```python
from build123d import *

# Parameters (mm, degrees)
ESQUISSE4_R           = 1.5
EXTRUSION3_DEPTH      = 25
ESQUISSE5_OUTSIDE_W   = 153.718
ESQUISSE5_OUTSIDE_H   = 153.718
ESQUISSE5_OUTSIDE_W_2 = 71
ESQUISSE5_OUTSIDE_H_2 = 48
EXTRUSION4_DEPTH      = 13
ESQUISSE6_R           = 2
EXTRUSION5_DEPTH      = 10
ESQUISSE7_R           = 2
EXTRUSION6_DEPTH      = 10


with BuildPart() as part:
    # Esquisse1 → Révolution1 (revolve)
    with BuildSketch(Plane.XY):
        Polygon((19, -12), (59, -12), (59, 0), (15, 0), (15, -20), (9, -20), (9, -24), (19, -24), align=None)
    revolve(axis=Axis((0, 0, 0), (0, -1, 0)))

    # Esquisse4 → Extrusion3 (cut, through all)
    with BuildSketch(Plane.XZ.offset(24)):
        with Locations((0, 13)):
            Circle(ESQUISSE4_R)
        with Locations((13, 0)):
            Circle(ESQUISSE4_R)
        with Locations((0, -13)):
            Circle(ESQUISSE4_R)
        with Locations((-13, 0)):
            Circle(ESQUISSE4_R)
    extrude(amount=-EXTRUSION3_DEPTH, mode=Mode.SUBTRACT)

    # Esquisse5 outside → Extrusion4 (cut, through all)
    with BuildSketch(Plane.XZ.offset(12)):
        Rectangle(ESQUISSE5_OUTSIDE_W, ESQUISSE5_OUTSIDE_H)
        Rectangle(ESQUISSE5_OUTSIDE_W_2, ESQUISSE5_OUTSIDE_H_2, mode=Mode.SUBTRACT)
    extrude(amount=-EXTRUSION4_DEPTH, mode=Mode.SUBTRACT)

    # Esquisse6 → Extrusion5 (cut)
    with BuildSketch(Plane(origin=(35.5, 0, 0), x_dir=(0, 0, -1), z_dir=(1, 0, 0))):
        with Locations((-15, -6)):
            Circle(ESQUISSE6_R)
        with Locations((15, -6)):
            Circle(ESQUISSE6_R)
    extrude(amount=-EXTRUSION5_DEPTH, mode=Mode.SUBTRACT)

    # Esquisse7 → Extrusion6 (cut)
    with BuildSketch(Plane.ZY.offset(35.5)):
        with Locations((15, -6)):
            Circle(ESQUISSE7_R)
        with Locations((-15, -6)):
            Circle(ESQUISSE7_R)
    extrude(amount=-EXTRUSION6_DEPTH, mode=Mode.SUBTRACT)


solid = part.part
```
The model under review builds one solid part; all positions refer to its coordinate system, in mm. A direction names the side the tool comes from. Round coordinates to 2 decimals unless told otherwise and drop trailing zeros. Order: outer loops, then holes, each group sorted by start corner. A loop starts at its lowest first (then second) coordinate and runs counter-clockwise, first axis right, second up. Notation, with made-up numbers: (31, 55) -> (73, 55) arc R18 cw to (73, 73) -> close; hole circle Ø4 at (-4, 28.5). An arc over 180 degrees is marked (long way). Use a Markdown table: item, result.
Q1. We need section B-B on x = -13. Write out the cut boundary in (y, z), then the cut area to 3 significant figures.
Values:
| item | result |
|---|---|
| outline | (-24, -13.86) -> (-12, -13.86) -> (-12, -24) -> (0, -24) -> (0, -7.48) -> (-20, -7.48) -> (-20, -1.5) -> (-24, -1.5) -> close; (-24, 1.5) -> (-20, 1.5) -> (-20, 7.48) -> (0, 7.48) -> (0, 24) -> (-12, 24) -> (-12, 13.86) -> (-24, 13.86) -> close |
| area | 597 mm^2 |
Q2. We need section A-A on y = -6. Write out the cut boundary in (x, z), then the cut area to 3 significant figures.
Values:
| item | result |
|---|---|
| outline | (-35.5, -24) -> (35.5, -24) -> (35.5, -17) -> (25.5, -17) -> (25.5, -13) -> (35.5, -13) -> (35.5, 13) -> (25.5, 13) -> (25.5, 17) -> (35.5, 17) -> (35.5, 24) -> (-35.5, 24) -> (-35.5, 17) -> (-25.5, 17) -> (-25.5, 13) -> (-35.5, 13) -> (-35.5, -13) -> (-25.5, -13) -> (-25.5, -17) -> (-35.5, -17) -> close; hole circle Ø30 at (0, 0) |
| area | 2,540 mm^2 |
Q3. We need section C-C on z = 20.5. Write out the cut boundary in (x, y), then the cut area to 3 significant figures.
Values:
| item | result |
|---|---|
| outline | (-35.5, -12) -> (35.5, -12) -> (35.5, 0) -> (-35.5, 0) -> close |
| area | 852 mm^2 |
Q4. Mouldability with a two-part tool opening along Z and no side actions: class faces 1 (the cylindrical face through (-0.325, -22.028, 11.536)), 2 (the cylindrical face through (30.6, -7.2, 16.6)), 3 (the flat face through (-35.5, -6, 0)), 4 (the cylindrical face through (8.767, -17.916, -16.856)) as +Z half, -Z half, draft (parallel to the pull), parting line (faces both ways), or undercut.
Values:
| item | result |
|---|---|
| face 1 | undercut |
| face 2 | undercut |
| face 3 | draft |
| face 4 | parting line |
Q5. For line 1 (Z direction, x = 0, y = -22.35); line 2 (Z direction, x = 0, y = -14.5); line 3 (Y direction, x = 9, z = 6.5), list the stretches that pass through material, from the lowest coordinate up.
Values:
| item | result |
|---|---|
| line 1 | z = -19 to -14.5, -11.5 to -9, 9 to 11.5, 14.5 to 19 |
| line 2 | z = -19 to -15, 15 to 19 |
| line 3 | y = -24 to -20 |
Q6. We need section D-D on y = -11. Write out the cut boundary in (x, z).
Values:
| item | result |
|---|---|
| outline | (-35.5, -24) -> (35.5, -24) -> (35.5, 24) -> (-35.5, 24) -> close; hole circle Ø30 at (0, 0) |
Q7. Clearance check with flat-ended pins moving along their axes: P1, Ø3.5, axis at x = 0, z = -13, coming from the +Y side; P2, Ø1.2, axis at y = -6, z = 14.5, coming from the -X side; P3, Ø2.5, axis at y = -6, z = -15, coming from the +X side. State where each tip first meets the part, or that it passes through.
Values:
| item | result |
|---|---|
| P1 | stops at y = -20 |
| P2 | stops at x = -25.5 |
| P3 | stops at x = 25.5 |
Q8. Tool access review of faces 5 (the flat face through (16.3, -12, -10.3)), 6 (the flat face through (25.5, -6, 15)), 7 (the flat face through (6.5, -20, -6.5)): name each direction out of +Z, -Z, +X, -X, +Y, -Y from which nothing blocks a thin tool from reaching the whole face with its end or side.
Values:
| item | result |
|---|---|
| face 5 | -Y |
| face 6 | +X |
| face 7 | +Y |
